from build123d import *

# Parameters (mm, degrees)
F0_W     = 20
F0_H     = 30
F0_W_2   = 10
F1_DEPTH = 10
F2_DEPTH = 20
F3_SIZE2 = 10
F3_SIZE  = 10
F4_SIZE2 = 10
F4_SIZE  = 10


with BuildPart() as f1:
    # F0 (on Top) → F1 (new body)
    with BuildSketch(Plane.XY):
        with Locations((10, 15)):
            Rectangle(F0_W, F0_H)
        Polygon((20, 30), (20, 0), (30, 0), (30, 30), (30, 40), (0, 40), (0, 30), align=None)
        with Locations((35, 15)):
            Rectangle(F0_W_2, F0_H)
    extrude(amount=-F1_DEPTH)

    # F0 (on Top) → F2 (join)
    with BuildSketch(Plane.XY):
        with Locations((10, 15)):
            Rectangle(F0_W, F0_H)
    extrude(amount=F2_DEPTH)

    # F3
    f3_edges = [f1.edges().sort_by_distance(p)[0] for p in [
        (10, 0, 20),
    ]]
    chamfer(f3_edges, length=F3_SIZE, length2=F3_SIZE2)

    # F4
    f4_edges = [f1.edges().sort_by_distance(p)[0] for p in [
        (40, 0, -5),
    ]]
    chamfer(f4_edges, length=F4_SIZE, length2=F4_SIZE2)


solid = f1.part
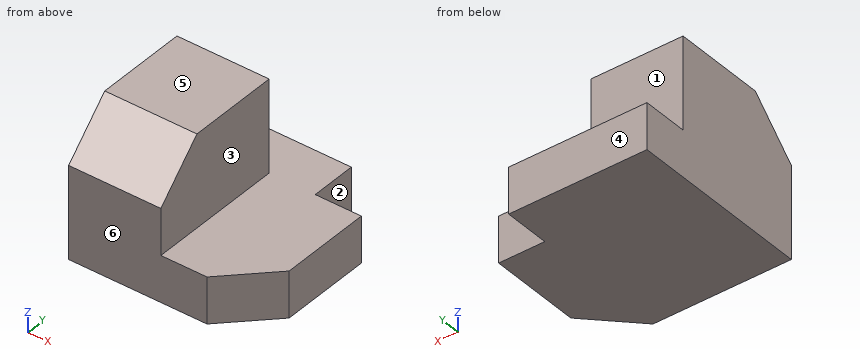
For this review, take the finished solid that the model builds, in its own axes (mm). Face numbers are marked on the shaded views. A direction names the side the tool comes from. Round coordinates to 2 decimals unless told otherwise and drop trailing zeros. Write each loop counter-clockwise with the first axis right and the second up, starting at its lowest first coordinate (ties: lowest second). Pieces come first, ordered by that corner, then holes. Notation, with made-up numbers: (81.5, 42.25) -> (118.5, 42.25) arc R20 ccw to (118.5, 57.25) -> close; hole circle Ø10 at (1, 25). An arc over 180 degrees is marked (long way). Use CSV: the item, a comma, the result in double quotes.
(1) Consider section A-A, the plane x = 7. Give the boundary of the cut face in (y, z), plus the area to 3 significant figures.
Computed values:
outline,"(0, -10) -> (40, -10) -> (40, 0) -> (30, 0) -> (30, 20) -> (10, 20) -> (0, 10) -> close"
area,"950 mm²"
(2) To check wall thickness, follow L1, parallel to X at y = 15, z = 15.5; L2, parallel to X at y = 33.5, z = -4.25. State the ranges of each line that lie inside material, in increasing order. Write a range as [from, to].
Computed values:
L1,"[0, 20]"
L2,"[0, 30]"
(3) Draft analysis for pull direction Y (two halves, no side actions). For the marked faces 4, 5 and 6, state which applies: +Y half, -Y half, draft (parallel to the pull), parting line (faces both ways), or undercut.
Computed values:
face 4,"+Y half"
face 5,"draft"
face 6,"-Y half"
(4) Consider section B-B, the plane y = 3. Give the boundary of the cut face in (x, z), plus the area to 3 significant figures.
Computed values:
outline,"(0, -10) -> (33, -10) -> (33, 0) -> (20, 0) -> (20, 13) -> (0, 13) -> close"
area,"590 mm²"
(5) Consider section D-D, the plane x = 36. Give the boundary of the cut face in (y, z).
Computed values:
outline,"(6, -10) -> (30, -10) -> (30, 0) -> (6, 0) -> close"
(6) Consider section C-C, the plane z = -3.5. Give the boundary of the cut face in (x, y).
Computed values:
outline,"(0, 0) -> (30, 0) -> (40, 10) -> (40, 30) -> (30, 30) -> (30, 40) -> (0, 40) -> close"
(7) For the marked faces 1, 2 and 3, list the 3-axis set-ups (+Z, -Z, +X, -X, +Y, -Y) from which the entire face can be reached by the end or side of a thin tool; tool diameter is ignored.
Computed values:
face 1,"+Z, +X, -X, +Y"
face 2,"+Z, -Z, +X, +Y"
face 3,"+Z, +X, +Y, -Y"
(8) Clearance check with flat-ended pins moving along their axes: P1, Ø6, axis at x = 32, y = 4, coming from the +Z side; P2, Ø8, axis at y = 36, z = -5, coming from the +X side; P3, Ø16, axis at x = 8.5, z = 12.5, coming from the +Y side. State where each tip first meets the part, or that it passes through.
Computed values:
P1,"z = 0"
P2,"x = 30"
P3,"y = 30"
